from build123d import *

# Parameters (mm, degrees)
BOSS_EXTRUDE1_DEPTH = 15
SKETCH4_R           = 7.5
CUT_EXTRUDE1_DEPTH  = 128.47548784


with BuildPart() as part:
    # Sketch1 → Boss-Extrude1 (new body)
    with BuildSketch(Plane.XY):
        with BuildLine():
            Line((-105, -20), (105, -20))
            ThreePointArc((105, -20), (125, 0), (105, 20))
            Line((105, 20), (-105, 20))
            ThreePointArc((-105, 20), (-125, 0), (-105, -20))
        make_face()
    extrude(amount=BOSS_EXTRUDE1_DEPTH)

    # Sketch4 → Cut-Extrude1 (cut, through all)
    with BuildSketch(Plane.XY.offset(15)):
        with Locations((105, 0)):
            Circle(SKETCH4_R)
    cut_extrude1 = extrude(amount=-CUT_EXTRUDE1_DEPTH, mode=Mode.SUBTRACT)

    # Mirror1: Cut-Extrude1 across plane
    add(cut_extrude1.mirror(Plane(origin=(0, 0, 0), x_dir=(0, 0, 1), z_dir=(1, 0, 0))), mode=Mode.SUBTRACT)


solid = part.part
The model under review builds one solid part; all positions refer to its coordinate system, in mm. Give positions to 0.01 mm unless a question says otherwise; leave off trailing zeros. Order: outer loops, then holes, each group sorted by start corner. A loop starts at its lowest first (then second) coordinate and runs counter-clockwise, first axis right, second up. Notation, with made-up numbers: M 53.5,10.5 L 107.5,10.5 A10 cw 107.5,24.5 Z; hole C 6.5,51 d5. An arc over 180 degrees is marked long. One line per question, with ' | ' between items. Start each with the question number.
1) Mouldability with a two-part tool opening along Y and no side actions: class faces 1 (the face through (1, 20, 7)), 2 (the face through (-112.154, 2.253, 7.605)), 3 (the face through (-2, 0, 15)) as pulls with the +Y half, pulls with the -Y half, needs draft (parallel to the pull), parting line crosses it, or undercut.
2) Consider section B-B, the plane y = 0. Give the boundary of the cut face in (x, z), then the cut area to 3 significant figures.
3) Consider section A-A, the plane x = -101. Give the boundary of the cut face in (y, z).
4) Consider section C-C, the plane z = 3. Give the boundary of the cut face in (x, y).
5) Wall thickness on L1, parallel to X at y = -5, z = 5; L2, parallel to Y at x = -105, z = 9; L3, parallel to X at y = 3.5, z = 9: over which ranges is each line inside the solid? List them lowest first. Write a range as from..to.
6) Clearance check with flat-ended pins moving along their axes: P1, Ø2, axis at y = -13, z = 8, coming from the -X side; P2, Ø5, axis at y = -2, z = 8.5, coming from the -X side; P3, Ø2, axis at y = 7, z = 12, coming from the -X side. State where each tip first meets the part, or that it passes through.
7) Consider section D-D, the plane y = 15. Give the boundary of the cut face in (x, z), then the cut area to 3 significant figures.
Found:
1) face 1: pulls with the +Y half | face 2: undercut | face 3: needs draft
2) outline: M -125,0 L -112.5,0 L -112.5,15 L -125,15 Z; M -97.5,0 L 97.5,0 L 97.5,15 L -97.5,15 Z; M 112.5,0 L 125,0 L 125,15 L 112.5,15 Z | area: 3,300 mm²
3) outline: M -20,0 L -6.34,0 L -6.34,15 L -20,15 Z; M 6.34,0 L 20,0 L 20,15 L 6.34,15 Z
4) outline: M -105,-20 L 105,-20 A20 ccw 105,20 L -105,20 A20 ccw Z; hole C -105,0 d15; hole C 105,0 d15
5) L1: x = -124.36..-110.59, -99.41..99.41, 110.59..124.36 | L2: y = -20..-7.5, 7.5..20 | L3: x = -124.69..-111.63, -98.37..98.37, 111.63..124.69
6) P1: stops at x = -121 | P2: stops at x = -125 | P3: stops at x = -124.08
7) outline: M -118.23,0 L 118.23,0 L 118.23,15 L -118.23,15 Z | area: 3,550 mm²
